Read the model definition and answer for the solid it produces. Units are mm, in the model's axes. A direction names the side the tool comes from. Coordinates: 2 decimals unless noted, no trailing zeros. Write each loop counter-clockwise with the first axis right and the second up, starting at its lowest first coordinate (ties: lowest second). Pieces come first, ordered by that corner, then holes.
(1) Straight lines are drawn through the part: line 1 along Y through (x, z) = (2, 3.9); line 2 along X through (y, z) = (3, 2.25); line 3 along Z through (x, y) = (8.5, -8.75). For each, find the intervals that lie inside material, in ascending order.
(2) The part is cut by section B-B, the plane z = 0.55. Determine the outline of the cut face in (x, y).
(3) The part is cut by section C-C, the plane x = 23. Determine the outline of the cut face in (y, z).
(4) Determine the mould class of faces 1 (the flat face through (15.5, 1.8, 2.5)), 2 (the flat face through (7, 2, 3)), 3 (the cylindrical face through (22.263, -3.324, 4.414)), 4 (the cylindrical face through (0.285, -0.301, 2.738)) for opening direction X: pulls with the +X half, pulls with the -X half, needs draft (parallel to the pull), parting line crosses it, or undercut.
(5) Which of the six approach directions +Z, -Z, +X, -X, +Y, -Y give full straight-line access (tool end or side, diameter ignored) to faces 5 (the flat face through (21.5, -12, 3)), 6 (the flat face through (18, -12, 3.3)), 7 (the flat face through (7, 2, 2))?
(6) The part is cut by section A-A, the plane y = -10.25. Determine the outline of the cut face in (x, z), and give its area (3 significant figures).
(7) Given pin 1 (1.3 mm diameter, centred on y = -10.5, z = 2.5, fed in from +X); pin 2 (0.5 mm diameter, centred on y = 2, z = 2.5, fed in from +X); pin 3 (3.5 mm diameter, centred on x = 8, y = -14, fed in from -Z), each flat-ended and moving along its own axis, determine where each tip first touches the part or whether it passes through.
(8) The part is cut by section D-D, the plane y = 1.5. Determine the outline of the cut face in (x, z), and give its area (3 significant figures).
```python
from build123d import *

# Parameters (mm, degrees)
SKETCH_1_W          = 25
SKETCH_1_H          = 8
EXTRUDE_1_DEPTH     = 5.4
SKETCH_2_W          = 7
SKETCH_2_H          = 1.2
EXTRUDE_2_DEPTH     = 9
SKETCH_3_W          = 5
SKETCH_3_H          = 1
EXTRUDE_3_DEPTH     = 4
CHAMFER_2_SIZE      = 0.4
CHAMFER_3_SIZE      = 0.4
SKETCH_4_R          = 1
CUT_EXTRUDE_1_DEPTH = 2
FILLET_1_R          = 1


with BuildPart() as part:
    # 草图1 → 凸台-拉伸1 (new body)
    with BuildSketch(Plane.XY):
        with Locations((12.5, -4)):
            Rectangle(SKETCH_1_W, SKETCH_1_H)
    extrude(amount=EXTRUDE_1_DEPTH)

    # 草图2 → 凸台-拉伸2 (add)
    with BuildSketch(Plane.XZ.offset(8)):
        with Locations((7, 2.7)):
            Rectangle(SKETCH_2_W, SKETCH_2_H)
        with Locations((18, 2.7)):
            Rectangle(SKETCH_2_W, SKETCH_2_H)
    extrude(amount=EXTRUDE_2_DEPTH)

    # 草图3 → 凸台-拉伸3 (add)
    with BuildSketch(Plane(origin=(0, 0, 0), x_dir=(1, 0, 0), z_dir=(0, 1, 0))):
        with Locations((7, -2.5)):
            Rectangle(SKETCH_3_W, SKETCH_3_H)
        with Locations((18, -2.5)):
            Rectangle(SKETCH_3_W, SKETCH_3_H)
    extrude(amount=EXTRUDE_3_DEPTH)

    # 倒角2
    chamfer_2_edges = [part.edges().sort_by_distance(p)[0] for p in [
        (3.5, -17, 2.7),
        (10.5, -17, 2.7),
        (14.5, -17, 2.7),
        (21.5, -17, 2.7),
        (4.5, 4, 2.5),
        (9.5, 4, 2.5),
        (15.5, 4, 2.5),
        (20.5, 4, 2.5),
    ]]
    chamfer(chamfer_2_edges, length=CHAMFER_2_SIZE)

    # 倒角3
    chamfer_3_edges = [part.edges().sort_by_distance(p)[0] for p in [
        (7, 4, 2),
        (7, 4, 3),
        (18, 4, 2),
        (18, 4, 3),
        (18, -17, 2.1),
        (18, -17, 3.3),
        (7, -17, 2.1),
        (7, -17, 3.3),
    ]]
    chamfer(chamfer_3_edges, length=CHAMFER_3_SIZE)

    # 草图4 → 切除-拉伸1 (cut)
    with BuildSketch(Plane.XY.offset(5.4)):
        with Locations((2, -4)):
            Circle(SKETCH_4_R)
        with Locations((23, -4)):
            Circle(SKETCH_4_R)
    extrude(amount=-CUT_EXTRUDE_1_DEPTH, mode=Mode.SUBTRACT)

    # 圆角1
    fillet_1_edges = [part.edges().sort_by_distance(p)[0] for p in [
        (0, 0, 2.7),
        (25, 0, 2.7),
        (25, -8, 2.7),
        (0, -8, 2.7),
    ]]
    fillet(fillet_1_edges, radius=FILLET_1_R)


solid = part.part
```
Computed:
1. line 1: y = -8 to -5, -3 to 0
1. line 2: x = 4.5 to 9.5, 15.5 to 20.5
1. line 3: z = 2.1 to 3.3
2. outline: (0, -7) arc R1 ccw to (1, -8) - (24, -8) arc R1 ccw to (25, -7) - (25, -1) arc R1 ccw to (24, 0) - (1, 0) arc R1 ccw to (0, -1) - close
3. outline: (-8, 0) - (0, 0) - (0, 5.4) - (-3, 5.4) - (-3, 3.4) - (-5, 3.4) - (-5, 5.4) - (-8, 5.4) - close
4. face 1: undercut
4. face 2: needs draft
4. face 3: undercut
4. face 4: pulls with the -X half
5. face 5: +Z, -Z, +X, -Y
5. face 6: +Z, +X, -X, -Y
5. face 7: -Z, +X, -X, +Y
6. outline: (3.5, 2.1) - (10.5, 2.1) - (10.5, 3.3) - (3.5, 3.3) - close; (14.5, 2.1) - (21.5, 2.1) - (21.5, 3.3) - (14.5, 3.3) - close
6. area: 16.8 mm2
7. pin 1: stops at x = 21.5
7. pin 2: stops at x = 20.5
7. pin 3: stops at z = 2.1
8. outline: (4.5, 2) - (9.5, 2) - (9.5, 3) - (4.5, 3) - close; (15.5, 2) - (20.5, 2) - (20.5, 3) - (15.5, 3) - close
8. area: 10.0 mm2
